```python
from build123d import *

# Parameters (mm, degrees)
SKETCH2_W               = 177.8
SKETCH2_H               = 152.4
BOSS_EXTRUDE1_DEPTH     = 50.8
SHELL2_T                = 2.54
BOSS_EXTRUDE3_START     = -33.02
BOSS_EXTRUDE3_OUTLINE_R = 12.7
BOSS_EXTRUDE3_DEPTH     = 30.48


# Read off the part's stored shape, not the designer's step: Boss-Extrude3
with BuildPart() as part:
    # Sketch2 → Boss-Extrude1 (new body)
    with BuildSketch(Plane.XY):
        Rectangle(SKETCH2_W, SKETCH2_H)
    extrude(amount=BOSS_EXTRUDE1_DEPTH)

    # Shell2
    shell2_openings = [part.faces().sort_by_distance(p)[0] for p in [
        (0, 0, 50.8),
    ]]
    offset(amount=SHELL2_T, openings=shell2_openings, kind=Kind.INTERSECTION)

    # Boss-Extrude3 outline → Boss-Extrude3 (add)
    with BuildSketch(Plane.XY.offset(BOSS_EXTRUDE3_START)):
        with Locations((-63.5, -50.8)):
            Circle(BOSS_EXTRUDE3_OUTLINE_R)
        with Locations((63.5, -50.8)):
            Circle(BOSS_EXTRUDE3_OUTLINE_R)
        with Locations((63.5, 50.8)):
            Circle(BOSS_EXTRUDE3_OUTLINE_R)
        with Locations((-63.5, 50.8)):
            Circle(BOSS_EXTRUDE3_OUTLINE_R)
    extrude(amount=BOSS_EXTRUDE3_DEPTH)


solid = part.part
```
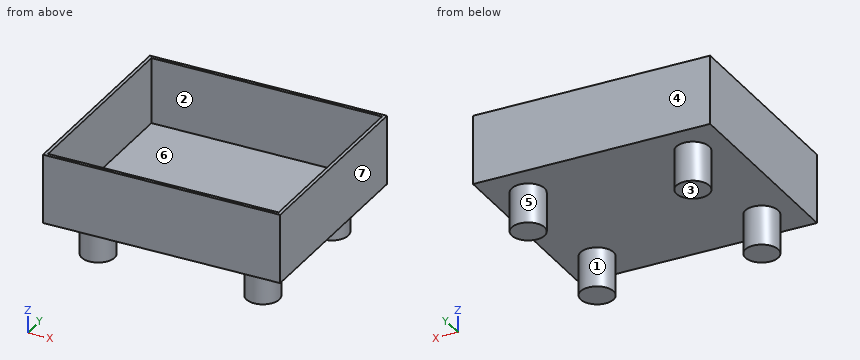
For this review, take the finished solid that the model builds, in its own axes (mm). Face numbers are marked on the shaded views. A direction names the side the tool comes from. Coordinates: 2 decimals unless noted, no trailing zeros. Loops run counter-clockwise (first coordinate to the right, second up) from the corner with the lowest first, then second, coordinate; pieces in that order, holes last.
1. For the marked faces 1, 2 and 3, list the 3-axis set-ups (+Z, -Z, +X, -X, +Y, -Y) from which the entire face can be reached by the end or side of a thin tool; tool diameter is ignored.
2. For line 1 (X direction, y = 68, z = 27); line 2 (Y direction, x = 70.5, z = 45.5); line 3 (Z direction, x = 43.5, y = -20.5), list the stretches that pass through material, from the lowest coordinate up.
3. Add section C-C, the plane z = 42. Give the boundary of the cut face in (x, y), then the cut area to 3 significant figures.
4. Mouldability with a two-part tool opening along Y and no side actions: class the marked faces 4, 5, 6 and 7 as +Y half, -Y half, draft (parallel to the pull), parting line (faces both ways), or undercut.
5. Add section B-B, the plane y = 28. Give the boundary of the cut face in (x, z), then the cut area to 3 significant figures.
6. Add section A-A, the plane x = 17.5. Give the boundary of the cut face in (y, z).
7. Add section D-D, the plane z = -18. Give the boundary of the cut face in (x, y).
8. Insertion check: P1, Ø8, axis at x = -43.5, y = 40.5, coming from the -Z side; P2, Ø10, axis at x = -52.5, y = 43, coming from the +Z side. Each pin has a flat end and moves straight along its axis. Give the tip position at first contact, or say it passes through.
Result:
1. face 1: -Z
1. face 2: +Z
1. face 3: -Z, +X, -X, +Y, -Y
2. line 1: x = -91.44 to -88.9, 88.9 to 91.44
2. line 2: y = -78.74 to -76.2, 76.2 to 78.74
2. line 3: z = -2.54 to 0
3. outline: (-91.44, -78.74) - (91.44, -78.74) - (91.44, 78.74) - (-91.44, 78.74) - close; hole (-88.9, -76.2) - (88.9, -76.2) - (88.9, 76.2) - (-88.9, 76.2) - close
3. area: 1,700 mm2
4. face 4: +Y half
4. face 5: undercut
4. face 6: undercut
4. face 7: draft
5. outline: (-91.44, -2.54) - (91.44, -2.54) - (91.44, 50.8) - (88.9, 50.8) - (88.9, 0) - (-88.9, 0) - (-88.9, 50.8) - (-91.44, 50.8) - close
5. area: 723 mm2
6. outline: (-78.74, -2.54) - (78.74, -2.54) - (78.74, 50.8) - (76.2, 50.8) - (76.2, 0) - (-76.2, 0) - (-76.2, 50.8) - (-78.74, 50.8) - close
7. outline: circle Ø25.4 at (-63.5, -50.8); circle Ø25.4 at (-63.5, 50.8); circle Ø25.4 at (63.5, -50.8); circle Ø25.4 at (63.5, 50.8)
8. P1: stops at z = -2.54
8. P2: stops at z = 0
